from build123d import *

# Parameters (mm, degrees)
CUT_EXTRUDE1_START = -10.16
SKETCH2_R          = 79.756
SKETCH2_R_2        = 76.2
CUT_EXTRUDE1_DEPTH = 10.16
FILLET1_R          = 1.5875


with BuildPart() as part:
    # Sketch1 → Revolve1 (revolve)
    with BuildSketch(Plane.XY, mode=Mode.PRIVATE) as revolve1_sk:
        Polygon((-83.82, -19.330547638), (-83.82, -17.425547638), (-82.296, -17.425547638), (-82.296, -7.265547638), (-76.2, -7.265547638), (-76.2, -17.425547638), (-76.2, -19.330547638), align=None)
    revolve(revolve1_sk.sketch.rotate(Axis((0, 0, 0), (0, 1, 0)), 270), axis=Axis((0, 0, 0), (0, 1, 0)))

    # Sketch2 → Cut-Extrude1 (cut)
    with BuildSketch(Plane(origin=(0, -7.265547638, 0), x_dir=(1, 0, 0), z_dir=(0, 1, 0)).offset(CUT_EXTRUDE1_START)):
        with Locations(Location((0, 0, 0), (0, 0, 270))):
            Circle(SKETCH2_R)
        with Locations(Location((0, 0, 0), (0, 0, 90))):
            Circle(SKETCH2_R_2, mode=Mode.SUBTRACT)
    extrude(amount=CUT_EXTRUDE1_DEPTH, mode=Mode.SUBTRACT)

    # Fillet1
    fillet1_edges = [part.edges().sort_by_distance(p)[0] for p in [
        (0, -17.425547638, -79.756),
    ]]
    fillet(fillet1_edges, radius=FILLET1_R)


solid = part.part
Read the model definition and answer for the solid it produces. Units are mm, in the model's axes. A direction names the side the tool comes from. Coordinates: 2 decimals unless noted, no trailing zeros. Write each loop counter-clockwise with the first axis right and the second up, starting at its lowest first coordinate (ties: lowest second). Pieces come first, ordered by that corner, then holes. Notation, with made-up numbers: M 63.5,14.5 L 94.5,14.5 A11 ccw 94.5,20.5 Z; hole C -6,23.25 d10. An arc over 180 degrees is marked long. Use a Markdown table: item, result.
Q1. Straight lines are drawn through the part: L1, parallel to X at y = -18.4, z = 0; L2, parallel to X at y = -9.75, z = 0; L3, parallel to Z at x = 27.5, y = -7.75 (3 decimals). For each, find the intervals that lie inside material, in ascending order. Write a range as [from, to].
Answer block:
| item | result |
|---|---|
| L1 | x = [-83.82, -76.2], [76.2, 83.82] |
| L2 | x = [-82.3, -79.76], [79.76, 82.3] |
| L3 | z = [-77.565, -74.865], [74.865, 77.565] |
Q2. The part is cut by section B-B, the plane x = 0. Write down the section's boundary in (y, z) (1 decimal).
Answer block:
| item | result |
|---|---|
| outline | M -19.3,-83.8 L -17.4,-83.8 L -17.4,-82.3 L -7.3,-82.3 L -7.3,-79.8 L -15.8,-79.8 A1.6 cw -17.4,-78.2 L -17.4,-76.2 L -19.3,-76.2 Z; M -19.3,76.2 L -17.4,76.2 L -17.4,78.2 A1.6 cw -15.8,79.8 L -7.3,79.8 L -7.3,82.3 L -17.4,82.3 L -17.4,83.8 L -19.3,83.8 Z |
Q3. The part is cut by section A-A, the plane z = 0. Write down the section's boundary in (x, y) (1 decimal), then the cut area to 3 significant figures.
Answer block:
| item | result |
|---|---|
| outline | M -83.8,-19.3 L -76.2,-19.3 L -76.2,-17.4 L -78.2,-17.4 A1.6 cw -79.8,-15.8 L -79.8,-7.3 L -82.3,-7.3 L -82.3,-17.4 L -83.8,-17.4 Z; M 76.2,-19.3 L 83.8,-19.3 L 83.8,-17.4 L 82.3,-17.4 L 82.3,-7.3 L 79.8,-7.3 L 79.8,-15.8 A1.6 cw 78.2,-17.4 L 76.2,-17.4 Z |
| area | 81.7 mm2 |
Q4. The part is cut by section C-C, the plane y = -11.5. Write down the section's boundary in (x, z), then the cut area to 3 significant figures.
Answer block:
| item | result |
|---|---|
| outline | C 0,0 d164.59; hole C 0,0 d159.51 |
| area | 1,290 mm2 |
Q5. Which of the six approach directions +Z, -Z, +X, -X, +Y, -Y give full straight-line access (tool end or side, diameter ignored) to faces 4 (the face through (79.077, -11.612, -10.383)), 5 (the face through (46.367, -18.365, 60.47))?
Answer block:
| item | result |
|---|---|
| face 4 | +Y |
| face 5 | +Y, -Y |
Q6. Each of these flat-tipped pins is pushed along its axis until it touches: pin 1 Ø5 at (y, z) = (-17, -31) entering from +X; pin 2 Ø5 at (y, z) = (-14, 65.5) entering from -X; pin 3 Ø2 at (y, z) = (-15, 27.5) entering from -X. Where does it stop, or does it pass through?
Answer block:
| item | result |
|---|---|
| pin 1 | stops at x = 78.81 |
| pin 2 | stops at x = -52.95 |
| pin 3 | stops at x = -77.91 |
Q7. Determine the mould class of faces 1 (the face through (-75, -17.426, 17)), 2 (the face through (-81.596, -12.274, 10.713)), 3 (the face through (55, -17.426, -62)) for opening direction Z: released by +Z, released by -Z, zero draft, split by the parting line, or undercut.
Answer block:
| item | result |
|---|---|
| face 1 | undercut |
| face 2 | split by the parting line |
| face 3 | zero draft |
